```python
from build123d import *

# Parameters (mm, degrees)
PAD_DEPTH    = 14
PAD001_DEPTH = 36
PAD002_DEPTH = 36
PAD003_DEPTH = 8
PAD004_DEPTH = 8
PAD005_DEPTH = 18
PAD006_DEPTH = 18


with BuildPart() as part:
    # Sketch → Pad (new body, symmetric)
    with BuildSketch(Plane.XY):
        with BuildLine():
            ThreePointArc((0, -15), (15, 0), (0, 15))
            ThreePointArc((0, 15), (-15, 0), (0, -15))
        make_face()
    extrude(amount=PAD_DEPTH, both=True)

    # Pad Face4 → Pad001 (add)
    with BuildSketch(Plane(origin=(0, 0, 14), x_dir=(0, 1, 0), z_dir=(0, 0, 1))):
        with BuildLine():
            ThreePointArc((-15, 0), (0, -15), (15, 0))
            ThreePointArc((15, 0), (0, 15), (-15, 0))
        make_face()
    extrude(amount=PAD001_DEPTH)

    # Pad001 Face3 → Pad002 (add)
    with BuildSketch(Plane(origin=(0, 0, -14), x_dir=(0, -1, 0), z_dir=(0, 0, -1))):
        with BuildLine():
            ThreePointArc((-15, 0), (0, -15), (15, 0))
            ThreePointArc((15, 0), (0, 15), (-15, 0))
        make_face()
    extrude(amount=PAD002_DEPTH)

    # Pad002 Face8 → Pad003 (add)
    with BuildSketch(Plane(origin=(0, 0, 50), x_dir=(0, 1, 0), z_dir=(0, 0, 1))):
        with BuildLine():
            ThreePointArc((-15, 0), (0, -15), (15, 0))
            ThreePointArc((15, 0), (0, 15), (-15, 0))
        make_face()
    extrude(amount=PAD003_DEPTH)

    # Pad003 Face7 → Pad004 (add)
    with BuildSketch(Plane(origin=(0, 0, -50), x_dir=(0, -1, 0), z_dir=(0, 0, -1))):
        with BuildLine():
            ThreePointArc((-15, 0), (0, -15), (15, 0))
            ThreePointArc((15, 0), (0, 15), (-15, 0))
        make_face()
    extrude(amount=PAD004_DEPTH)

    # Pad004 Face11 → Pad005 (add)
    with BuildSketch(Plane(origin=(0, 0, -58), x_dir=(0, -1, 0), z_dir=(0, 0, -1))):
        with BuildLine():
            ThreePointArc((-15, 0), (0, -15), (15, 0))
            ThreePointArc((15, 0), (0, 15), (-15, 0))
        make_face()
    extrude(amount=PAD005_DEPTH)

    # Pad005 Face12 → Pad006 (add)
    with BuildSketch(Plane(origin=(0, 0, 58), x_dir=(0, 1, 0), z_dir=(0, 0, 1))):
        with BuildLine():
            ThreePointArc((-15, 0), (0, -15), (15, 0))
            ThreePointArc((15, 0), (0, 15), (-15, 0))
        make_face()
    extrude(amount=PAD006_DEPTH)


solid = part.part
```
Part model, mm, in its own coordinate system. Give positions to 0.01 mm unless a question says otherwise; leave off trailing zeros. Write each loop counter-clockwise with the first axis right and the second up, starting at its lowest first coordinate (ties: lowest second). Pieces come first, ordered by that corner, then holes. Notation, with made-up numbers: (47, 31) -> (95, 31) arc R28 cw to (95, 63) -> close; hole circle Ø5 at (6.25, -15.5). An arc over 180 degrees is marked (long way). Put each result on its own line as item: value. Start each with the question number.
Item 1: Cut at A-A (z = 47.5). List the corners of the cut face in (x, y).
Item 2: Cut at B-B (y = 13). List the corners of the cut face in (x, z), then the cut area to 3 significant figures.
Item 3: Pin check, flat tips, straight feed: pin 1 Ø1.5 at (y, z) = (4.5, 9) entering from -X; pin 2 Ø6 at (x, z) = (10, 15) entering from +Y; pin 3 Ø2 at (y, z) = (10, 44.5) entering from +X. Stop position of each tip, or through.
Item 4: Wall check: L1, parallel to X at y = -0.5, z = 24; L2, parallel to X at y = 11, z = -36; L3, parallel to Y at x = -9.25, z = 2.5. Give the ranges that are in metal, low to high. Write a range as [from, to].
Answer list:
1. outline: circle Ø30 at (0, 0)
2. outline: (-7.48, -76) -> (7.48, -76) -> (7.48, 76) -> (-7.48, 76) -> close
2. area: 2,270 mm2
3. pin 1: stops at x = -14.52
3. pin 2: stops at y = 13.27
3. pin 3: stops at x = 12
4. L1: x = [-14.99, 14.99]
4. L2: x = [-10.2, 10.2]
4. L3: y = [-11.81, 11.81]
